```python
from build123d import *

# Parameters (mm, degrees)
SKETCH1_W          = 76.2
SKETCH1_H          = 73.025
EXTRUDE1_DEPTH     = 9.525
SKETCH8_R          = 3.175
SKETCH8_R_2        = 9.525
CUT_EXTRUDE5_DEPTH = 10.525


with BuildPart() as part:
    # Sketch1 → Extrude1 (new body)
    with BuildSketch(Plane(origin=(0, 0, 0), x_dir=(0, 0, -1), z_dir=(1, 0, 0))):
        with Locations((38.1, -36.5125)):
            Rectangle(SKETCH1_W, SKETCH1_H)
    extrude(amount=EXTRUDE1_DEPTH)

    # Sketch8 → Cut-Extrude5 (cut, through all)
    with BuildSketch(Plane.ZY):
        with Locations((-7.1374, -7.1374)):
            Circle(SKETCH8_R)
        with Locations((-69.0626, -7.1374)):
            Circle(SKETCH8_R)
        with Locations((-69.0626, -65.8876)):
            Circle(SKETCH8_R)
        with Locations((-7.1374, -65.8876)):
            Circle(SKETCH8_R)
        with Locations((-38.1, -34.925)):
            Circle(SKETCH8_R_2)
    extrude(amount=-CUT_EXTRUDE5_DEPTH, mode=Mode.SUBTRACT)


solid = part.part
```
The listing builds one solid part. Answer for the finished solid, in the listing's coordinates (mm). Give positions to 0.01 mm unless a question says otherwise; leave off trailing zeros. Write each loop counter-clockwise with the first axis right and the second up, starting at its lowest first coordinate (ties: lowest second). Pieces come first, ordered by that corner, then holes. Notation, with made-up numbers: M 59.25,71.25 L 91.25,71.25 A29 cw 91.25,108.25 Z; hole C 65.25,-7 d3. An arc over 180 degrees is marked long. Write each question's results on one line, items separated by ' | '.
Q1. Consider L1, parallel to Y at x = 1.5, z = -66.5 (3 decimals); L2, parallel to Z at x = 9.25, y = -63; L3, parallel to Z at x = 8.25, y = -5.5. Determine where each line is inside the solid, lowest interval first. Write a range as from..to.
Output values:
L1: -73.025..-67.762, -64.013..-9.012, -5.263..0 | L2: -76.2..-70.38, -67.74..-8.46, -5.82..0 | L3: -76.2..-71.78, -66.34..-9.86, -4.42..0
Q2. Section C-C, the plane y = -38 is taken. Write down the section's boundary in (x, z) (3 decimals).
Output values:
outline: M 0,-76.2 L 9.525,-76.2 L 9.525,-47.115 L 0,-47.115 Z; M 0,-29.085 L 9.525,-29.085 L 9.525,0 L 0,0 Z
Q3. For a pull along Z with two mould halves and no side action, classify faces 1 (the cylindrical face through (4.696, -32.064, -29.015)), 2 (the flat face through (5, -37, 0)), 3 (the flat face through (9.525, -44, -46)) as released by +Z, released by -Z, zero draft, split by the parting line, or undercut.
Output values:
face 1: undercut | face 2: released by +Z | face 3: zero draft
Q4. Section A-A, the plane z = -38.1 is taken. Write down the section's boundary in (x, y) (3 decimals).
Output values:
outline: M 0,-73.025 L 9.525,-73.025 L 9.525,-44.45 L 0,-44.45 Z; M 0,-25.4 L 9.525,-25.4 L 9.525,0 L 0,0 Z
Q5. Section B-B, the plane x = 8 is taken. Write down the section's boundary in (y, z) (3 decimals), then the cut area to 3 significant figures.
Output values:
outline: M -73.025,-76.2 L 0,-76.2 L 0,0 L -73.025,0 Z; hole C -65.888,-69.063 d6.35; hole C -65.888,-7.137 d6.35; hole C -34.925,-38.1 d19.05; hole C -7.137,-69.063 d6.35; hole C -7.137,-7.137 d6.35 | area: 5,150 mm2
Q6. A flat-ended cylindrical pin translates along its axis: P1, Ø5, axis at y = -7.14, z = -7.14, coming from the -X side. Find the tip coordinate at first contact, or state that the pin passes through.
Output values:
P1: through
